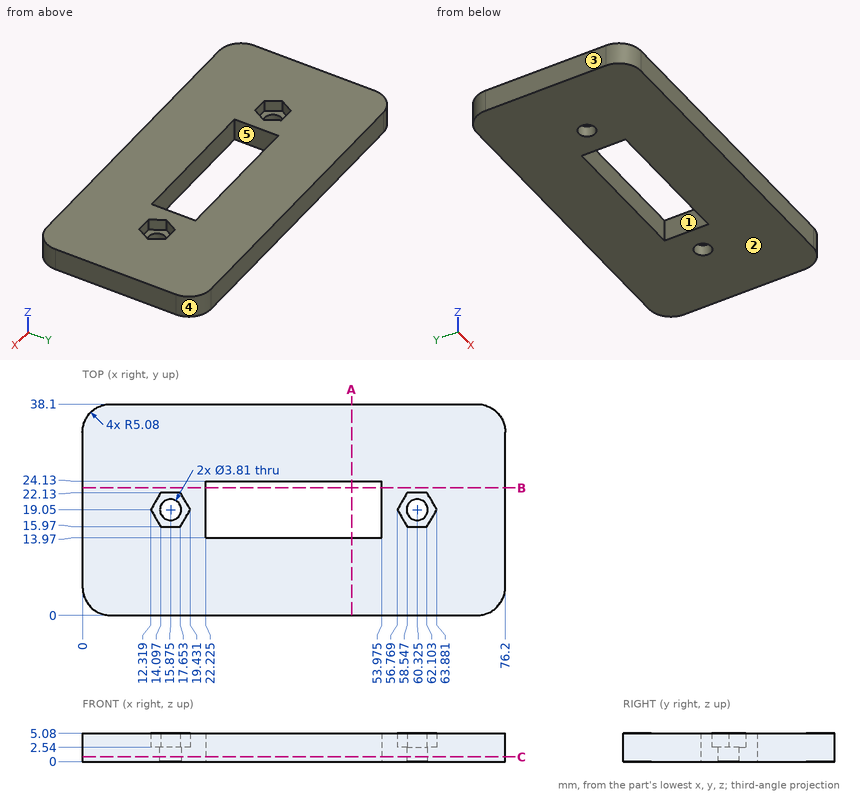
Could you check a few things on this drawing? It's one solid part, dimensions in mm from its lowest x, y, z. A direction names the side the tool comes from. Give positions to 0.01 mm unless a question says otherwise; leave off trailing zeros. Loops run counter-clockwise (first coordinate to the right, second up) from the corner with the lowest first, then second, coordinate; pieces in that order, holes last. Notation, with made-up numbers: (24.5, -6) -> (39.5, -6) arc R17 cw to (39.5, 3) -> close; hole circle Ø11 at (-15.5, 84.25). An arc over 180 degrees is marked (long way). Answer as CSV lines item,"result". Start each with the question number.
(1) If we section it at A-A on x = 48.5: Write out the boundary of the cut face in (y, z).
(2) I'm going to push flat-ended pins straight in: pin 1 Ø1 at (y, z) = (27.5, 4.5) entering from -X; pin 2 Ø4.5 at (x, y) = (60.325, 19.05) entering from +Z. Where does each tip first touch, or does it pass through?
(3) Which directions (+Z, -Z, +X, -X, +Y, -Y) give clear straight access to the entire face, cutting with the end or side of a thin tool? Please do the marked faces 4 and 5.
(4) If we section it at C-C on z = 0.85: Count the separate pieces of the cut face and the enclosed holes in it, then the cut area to 3 significant figures.
(5) We'd pull the mould along X, two halves only. Please class the marked faces 1, 2 and 3: released by +X, released by -X, zero draft, split by the parting line, or undercut.
(6) If we section it at B-B on y = 23: Write out the boundary of the cut face in (x, z) (1 decimal).
(7) I need wall thicknesses on probe 1 along Y at (x, z) = (47.5, 2.4); probe 2 along X at (y, z) = (20, 3.9) (1 decimal); probe 3 along Y at (x, z) = (72, 1.8). Which ranges of each line are inside material? Lowest first, please.
Computed:
1,outline,"(0, 0) -> (13.97, 0) -> (13.97, 5.08) -> (0, 5.08) -> close; (24.13, 0) -> (38.1, 0) -> (38.1, 5.08) -> (24.13, 5.08) -> close"
2,pin 1,"stops at x = 0"
2,pin 2,"stops at z = 2.54"
3,face 4,"+Z, -Z, +X, +Y"
3,face 5,"+Z, -Z"
4,separate pieces,"1"
4,enclosed holes,"3"
4,area,"2,540 mm2"
5,face 1,"undercut"
5,face 2,"zero draft"
5,face 3,"released by -X"
6,outline,"(0, 0) -> (22.2, 0) -> (22.2, 5.1) -> (0, 5.1) -> close; (54, 0) -> (76.2, 0) -> (76.2, 5.1) -> (54, 5.1) -> close"
7,probe 1,"y = 0 to 13.97, 24.13 to 38.1"
7,probe 2,"x = 0 to 12.9, 18.9 to 22.2, 54 to 57.3, 63.3 to 76.2"
7,probe 3,"y = 0.08 to 38.02"
